Could you check a few things on this model? Use its own coordinates, in mm. A direction names the side the tool comes from. Coordinates: 2 decimals unless noted, no trailing zeros. Loops run counter-clockwise (first coordinate to the right, second up) from the corner with the lowest first, then second, coordinate; pieces in that order, holes last.
from build123d import *

# Parameters (mm, degrees)
SKETCH3_W          = 6.35
SKETCH3_H          = 6.35
CUT_EXTRUDE1_DEPTH = 198.872684098


with BuildPart() as part:
    # Sketch2 → Revolve1 (revolve)
    with BuildSketch(Plane.XY, mode=Mode.PRIVATE) as revolve1_sk:
        Polygon((0, 0), (-28.575, 0), (-28.575, 190.5), (-29.845, 190.5), (-29.845, 193.04), (-30.734, 193.04), (-30.734, -6.35), (0, -6.35), align=None)
    revolve(revolve1_sk.sketch.rotate(Axis((0, -6.35, 0), (0, 1, 0)), 270), axis=Axis((0, -6.35, 0), (0, 1, 0)))

    # Sketch3 → Cut-Extrude1 (cut, through all)
    with BuildSketch(Plane(origin=(0, 0, 0), x_dir=(1, 0, 0), z_dir=(0, 1, 0))):
        Rectangle(SKETCH3_W, SKETCH3_H)
    extrude(amount=-CUT_EXTRUDE1_DEPTH, mode=Mode.SUBTRACT)


solid = part.part
(1) I need wall thicknesses on probe 1 along X at (y, z) = (127, 0) (3 decimals); probe 2 along Z at (x, y) = (0.5, 58); probe 3 along Y at (x, z) = (0.5, 26.5). Which ranges of each line are inside material? Lowest first, please.
Answers:
probe 1: x = -30.734 to -28.575, 28.575 to 30.734
probe 2: z = -30.73 to -28.57, 28.57 to 30.73
probe 3: y = -6.35 to 0
(2) Imagine slicing it at D-D, the plane x = 8.5. Write out the boundary of the cut face in (y, z), and give its area (3 significant figures).
Answers:
outline: (-6.35, -29.54) - (193.04, -29.54) - (193.04, -28.61) - (190.5, -28.61) - (190.5, -27.28) - (0, -27.28) - (0, 27.28) - (190.5, 27.28) - (190.5, 28.61) - (193.04, 28.61) - (193.04, 29.54) - (-6.35, 29.54) - close
area: 1,240 mm2
(3) We'd pull the mould along Z, two halves only. Please class faces 1 (the face through (29, 190.5, 0)), 2 (the face through (30.003, 91.949, 6.663)), 3 (the face through (6, -6.35, 0)), 4 (the face through (3.175, -3, 0)): +Z half, -Z half, draft (parallel to the pull), parting line (faces both ways), or undercut.
Answers:
face 1: undercut
face 2: parting line
face 3: draft
face 4: undercut
(4) Which directions (+Z, -Z, +X, -X, +Y, -Y) give clear straight access to the entire face, cutting with the end or side of a thin tool? Please do faces 5 (the face through (-30, 193.04, -5)), 6 (the face through (0, -3, 3.175)), 7 (the face through (-1.256, 96.584, 28.547)).
Answers:
face 5: +Z, -Z, +X, -X, +Y
face 6: +Y, -Y
face 7: +Y
(5) Imagine slicing it at C-C, the plane y = 63.5. Write out the boundary of the cut face in (x, z) (3 decimals), and give its area (3 significant figures).
Answers:
outline: circle Ø61.468 at (0, 0); hole circle Ø57.15 at (0, 0)
area: 402 mm2
(6) For pin 1 (3 mm diameter, centred on y = -4.5, z = -1.5, fed in from -X); pin 2 (5 mm diameter, centred on y = -2, z = -1, fed in from +X); pin 3 (8 mm diameter, centred on x = 12.5, z = -22.5, fed in from +Y), each with a flat end and sliding along its axis, tell me the tip position at first contact or that it passes through.
Answers:
pin 1: stops at x = -30.73
pin 2: stops at x = 30.73
pin 3: stops at y = 190.5
(7) Imagine slicing it at A-A, the plane z = 0. Write out the boundary of the cut face in (x, y) (3 decimals).
Answers:
outline: (-30.734, -6.35) - (-3.175, -6.35) - (-3.175, 0) - (-28.575, 0) - (-28.575, 190.5) - (-29.845, 190.5) - (-29.845, 193.04) - (-30.734, 193.04) - close; (3.175, -6.35) - (30.734, -6.35) - (30.734, 193.04) - (29.845, 193.04) - (29.845, 190.5) - (28.575, 190.5) - (28.575, 0) - (3.175, 0) - close
(8) Imagine slicing it at B-B, the plane x = 0. Write out the boundary of the cut face in (y, z) (3 decimals), and give its area (3 significant figures).
Answers:
outline: (-6.35, -30.734) - (193.04, -30.734) - (193.04, -29.845) - (190.5, -29.845) - (190.5, -28.575) - (0, -28.575) - (0, -3.175) - (-6.35, -3.175) - close; (-6.35, 3.175) - (0, 3.175) - (0, 28.575) - (190.5, 28.575) - (190.5, 29.845) - (193.04, 29.845) - (193.04, 30.734) - (-6.35, 30.734) - close
area: 1,180 mm2
